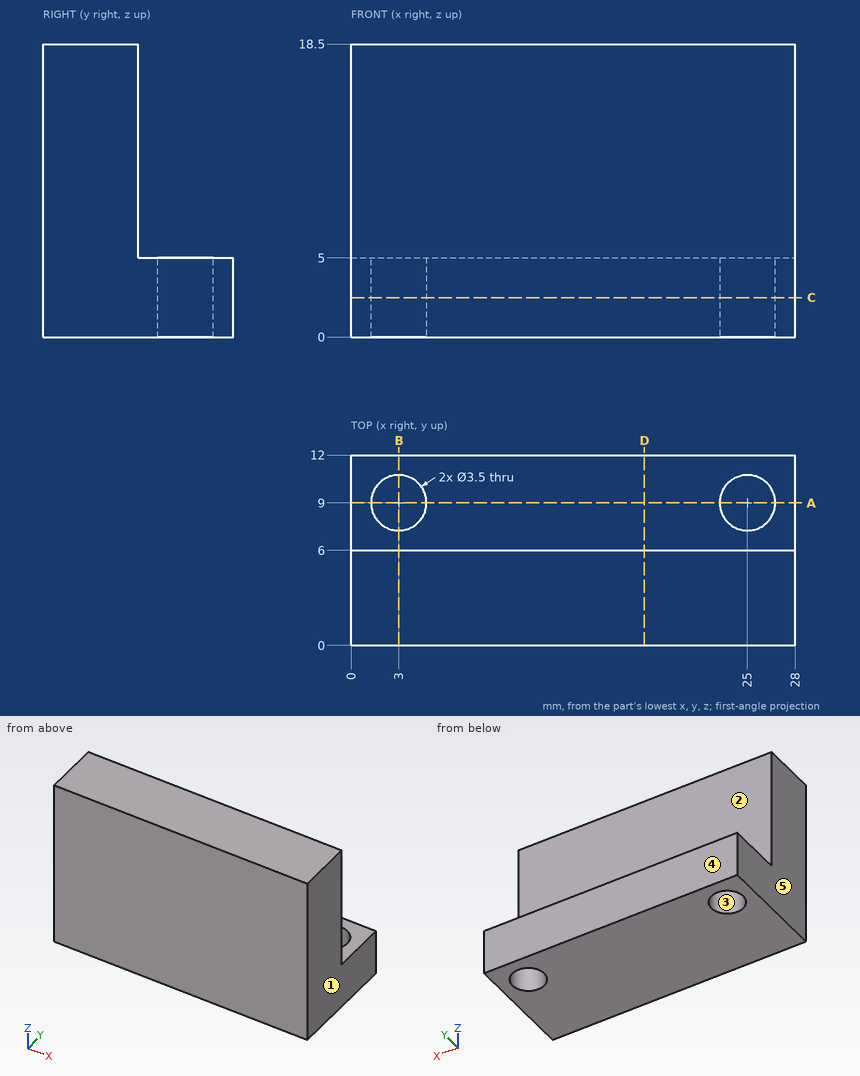
Input: dimensioned drawing with shaded views. Units: mm. Origin: part minimum x, y, z. A direction names the side the tool comes from. Coordinates: 2 decimals unless noted, no trailing zeros. Order: outer loops, then holes, each group sorted by start corner. A loop starts at its lowest first (then second) coordinate and runs counter-clockwise, first axis right, second up. Notation, with made-up numbers: (37.5, 15) -> (83.5, 15) arc R4 cw to (83.5, 21) -> close; hole circle Ø9 at (47, -33.75). An arc over 180 degrees is marked (long way). Use CSV: the item, a comma, the result in double quotes.
1) Section A-A on y = 9. Output: boundary loops of the cut face in (x, z).
Findings:
outline,"(0, 0) -> (1.25, 0) -> (1.25, 5) -> (0, 5) -> close; (4.75, 0) -> (23.25, 0) -> (23.25, 5) -> (4.75, 5) -> close; (26.75, 0) -> (28, 0) -> (28, 5) -> (26.75, 5) -> close"
2) Section B-B on x = 3. Output: boundary loops of the cut face in (y, z).
Findings:
outline,"(0, 0) -> (7.25, 0) -> (7.25, 5) -> (6, 5) -> (6, 18.5) -> (0, 18.5) -> close; (10.75, 0) -> (12, 0) -> (12, 5) -> (10.75, 5) -> close"
3) Pin query (flat end, axial travel): pin 1 Ø2 at (y, z) = (1.5, 5.5) entering from -X; pin 2 Ø1.5 at (x, y) = (16, 7.5) entering from +Z; pin 3 Ø11 at (x, z) = (13, 11) entering from +Y. Return the tip coordinate at first contact, or that it passes through.
Findings:
pin 1,"stops at x = 0"
pin 2,"stops at z = 5"
pin 3,"stops at y = 6"
4) Section D-D on x = 18.5. Output: boundary loops of the cut face in (y, z), then the cut area to 3 significant figures.
Findings:
outline,"(0, 0) -> (12, 0) -> (12, 5) -> (6, 5) -> (6, 18.5) -> (0, 18.5) -> close"
area,"141 mm^2"
5) Mould query, pull axis X, two halves, no side actions, for the marked faces 3, 4 and 5. Classes: +X half, -X half, draft (parallel to the pull), parting line (faces both ways), or undercut.
Findings:
face 3,"undercut"
face 4,"draft"
face 5,"-X half"
6) Line query: line 1 (Y direction, x = 25, z = 3.35); line 2 (Y direction, x = 17, z = 13.5); line 3 (Z direction, x = 19.25, y = 10.5). Output: solid intervals per line, ascending.
Findings:
line 1,"y = 0 to 7.25, 10.75 to 12"
line 2,"y = 0 to 6"
line 3,"z = 0 to 5"
7) Section C-C on z = 2.5. Output: boundary loops of the cut face in (x, y).
Findings:
outline,"(0, 0) -> (28, 0) -> (28, 12) -> (0, 12) -> close; hole circle Ø3.5 at (3, 9); hole circle Ø3.5 at (25, 9)"
8) Access query for the marked faces 1 and 2. Directions: +Z, -Z, +X, -X, +Y, -Y. A direction counts if a zero-diameter tool reaches every point of the face in a straight line with its end or side. Return the directions, or none.
Findings:
face 1,"+Z, -Z, +X, +Y, -Y"
face 2,"+Z, +X, -X, +Y"
